```python
from build123d import *

# Parameters (mm, degrees)
F0_W     = 50.8
F0_H     = 50.8
F1_DEPTH = 12.7
F2_W     = 50.8
F2_H     = 12.7
F3_DEPTH = 50.8
F5_DEPTH = 12.7


with BuildPart() as f1:
    # F0 (on Top) → F1 (new body)
    with BuildSketch(Plane.XY):
        Rectangle(F0_W, F0_H)
    extrude(amount=F1_DEPTH)

    # F2 (on Top) → F3 (join)
    with BuildSketch(Plane.XY):
        with Locations((0, 31.622227)):
            Rectangle(F2_W, F2_H)
    extrude(amount=F3_DEPTH)

    # F4 (on face) → F5 (cut)
    with BuildSketch(Plane.XZ.offset(-25.272227)):
        with BuildLine():
            ThreePointArc((0, 38.1), (-6.286179, 22.923821), (8.89, 29.21))
            ThreePointArc((8.89, 29.21), (6.286179, 35.496179), (0, 38.1))
        make_face()
    extrude(amount=-F5_DEPTH, mode=Mode.SUBTRACT)


solid = f1.part
```
Verification items for the finished model (mm, model axes). A direction names the side the tool comes from. Round coordinates to 2 decimals unless told otherwise and drop trailing zeros. Order: outer loops, then holes, each group sorted by start corner. A loop starts at its lowest first (then second) coordinate and runs counter-clockwise, first axis right, second up. Notation, with made-up numbers: (68, -30) - (123, -30) arc R22 cw to (123, -12) - close; hole circle Ø11 at (-38, -2.5). An arc over 180 degrees is marked (long way). Use CSV: the item, a comma, the result in double quotes. Start each with the question number.
1) Section check C-C, the plane x = 16.5. Record the cut outline in (y, z).
2) Section check B-B, the plane y = 28.5. Record the cut outline in (x, z).
3) Go/stop test with a flat-tipped pin: P1, Ø20.5, axis at x = 0, z = 29.21, coming from the -Y side. Record where the tip stops, or that it passes through.
4) Section check A-A, the plane x = -1.5. Record the cut outline in (y, z).
5) Thickness scan on L1, parallel to X at y = 30.75, z = 29.21; L2, parallel to Z at x = 17, y = 16; L3, parallel to Y at x = -19.5, z = 27.5. Record the ranges inside material, lowest first.
6) Section check D-D, the plane y = 6. Record the cut outline in (x, z), plus the area to 3 significant figures.
7) Access from +Z, -Z, +X, -X, +Y, -Y to the whole of each face (thin tool, end or side, straight path). Record for faces 1 (the flat face through (25.4, 20, 8)), 2 (the flat face through (0, 0, 12.7)).
Answers:
1,outline,"(-25.4, 0) - (37.97, 0) - (37.97, 50.8) - (25.27, 50.8) - (25.27, 12.7) - (-25.4, 12.7) - close"
2,outline,"(-25.4, 0) - (25.4, 0) - (25.4, 50.8) - (-25.4, 50.8) - close; hole (0, 38.1) arc R8.89 ccw (long way) to (8.89, 29.21) arc R8.89 ccw to start"
3,P1,"stops at y = 25.27"
4,outline,"(-25.4, 0) - (37.97, 0) - (37.97, 20.45) - (25.27, 20.45) - (25.27, 12.7) - (-25.4, 12.7) - close; (25.27, 37.97) - (37.97, 37.97) - (37.97, 50.8) - (25.27, 50.8) - close"
5,L1,"x = -25.4 to -8.89, 8.89 to 25.4"
5,L2,"z = 0 to 12.7"
5,L3,"y = 25.27 to 37.97"
6,outline,"(-25.4, 0) - (25.4, 0) - (25.4, 12.7) - (-25.4, 12.7) - close"
6,area,"645 mm²"
7,face 1,"+Z, -Z, +X, +Y, -Y"
7,face 2,"+Z, +X, -X, -Y"
